from build123d import *

# Parameters (mm, degrees)
BOSS_EXTRUDE1_DEPTH = 4.7625
SKETCH2_R           = 1.25
SKETCH2_W           = 10
SKETCH2_H           = 5
SKETCH2_W_2         = 8
SKETCH2_H_2         = 6
CUT_EXTRUDE1_DEPTH  = 5.7625


with BuildPart() as part:
    # Sketch1 → Boss-Extrude1 (new body)
    with BuildSketch(Plane.XY):
        Polygon((70.6, 40.2), (57.423529412, 29), (0, 29), (0, 0), (84, 0), (100, 29), (100, 40.2), align=None)
    extrude(amount=BOSS_EXTRUDE1_DEPTH)

    # Sketch2 → Cut-Extrude1 (cut, through all)
    with BuildSketch(Plane.XY.offset(4.7625)):
        with Locations((97.2, 37.4)):
            Circle(SKETCH2_R)
        with Locations((75.2, 37.4)):
            Circle(SKETCH2_R)
        with Locations((67.4, 31.1)):
            Circle(SKETCH2_R)
        with Locations((67.4, 9.1)):
            Circle(SKETCH2_R)
        with Locations((75.2, 2.8)):
            Circle(SKETCH2_R)
        with Locations((11, 26.2)):
            Circle(SKETCH2_R)
        with Locations((27, 26.2)):
            Circle(SKETCH2_R)
        with Locations((27, 2.8)):
            Circle(SKETCH2_R)
        with Locations((11, 2.8)):
            Circle(SKETCH2_R)
        with Locations((77.6, 29.7)):
            Rectangle(SKETCH2_W, SKETCH2_H)
        with Locations((77.6, 10.5)):
            Rectangle(SKETCH2_W, SKETCH2_H)
        with Locations((19, 20.5)):
            Rectangle(SKETCH2_W_2, SKETCH2_H_2)
        with Locations((19, 8.5)):
            Rectangle(SKETCH2_W_2, SKETCH2_H_2)
    extrude(amount=-CUT_EXTRUDE1_DEPTH, mode=Mode.SUBTRACT)


solid = part.part
Here's how the part is built. I have some questions about the finished solid (model axes, mm). A direction names the side the tool comes from. Coordinates: 2 decimals unless noted, no trailing zeros. Write each loop counter-clockwise with the first axis right and the second up, starting at its lowest first coordinate (ties: lowest second). Pieces come first, ordered by that corner, then holes. Notation, with made-up numbers: (-30, 37.5) - (-6, 37.5) arc R25 ccw to (-6, 54.5) - close; hole circle Ø11 at (-21.5, -1). An arc over 180 degrees is marked (long way). Use one line per item in the form item = value.
1) I'm going to push flat-ended pins straight in: P1, Ø1.5, axis at x = 75.2, y = 2.8, coming from the +Z side; P2, Ø2.5, axis at y = 10.5, z = 3.5, coming from the +X side; P3, Ø1.4, axis at x = 18.5, z = 2.5, coming from the +Y side. Where does each tip first touch, or does it pass through?
Solved:
P1 = through
P2 = 90.48
P3 = 29
2) Thinking about a two-plate mould opening in X: for faces 4 (the cylindrical face through (10.079, 3.645, 2.415)), 5 (the flat face through (72.6, 30, 2)), 6 (the flat face through (100, 35, 2)), 7 (the flat face through (0, 15, 2)), which applies, released by +X, released by -X, zero draft, split by the parting line, or undercut?
Solved:
face_4 = undercut
face_5 = undercut
face_6 = released by +X
face_7 = released by -X
3) Suppose I cut it at A-A, the plane x = 67.4. Write out the boundary of the cut face in (y, z), plus the area to 3 significant figures.
Solved:
outline = (0, 0) - (7.85, 0) - (7.85, 4.76) - (0, 4.76) - close; (10.35, 0) - (29.85, 0) - (29.85, 4.76) - (10.35, 4.76) - close; (32.35, 0) - (37.48, 0) - (37.48, 4.76) - (32.35, 4.76) - close
area = 155 mm2
4) Suppose I cut it at B-B, the plane z = 2.85. Give the number of separate pieces and of enclosed holes in the cut face, plus the area to 3 significant figures.
Solved:
separate_pieces = 1
enclosed_holes = 13
area = 2,830 mm2
5) On a 3-axis mill with a long thin cutter (end or side, diameter ignored), from which of +Z, -Z, +X, -X, +Y, -Y can I reach the whole of each face in a straight line? I mean faces 1 (the flat face through (82.6, 10, 2)), 2 (the flat face through (29, 29, 2)), 3 (the flat face through (41, 0, 2)). Say none if no direction works.
Solved:
face_1 = +Z, -Z
face_2 = +Z, -Z, -X, +Y
face_3 = +Z, -Z, +X, -X, -Y
6) Suppose I cut it at C-C, the plane y = 9.1. Write out the boundary of the cut face in (x, z), plus the area to 3 significant figures.
Solved:
outline = (0, 0) - (15, 0) - (15, 4.76) - (0, 4.76) - close; (23, 0) - (66.15, 0) - (66.15, 4.76) - (23, 4.76) - close; (68.65, 0) - (72.6, 0) - (72.6, 4.76) - (68.65, 4.76) - close; (82.6, 0) - (89.02, 0) - (89.02, 4.76) - (82.6, 4.76) - close
area = 326 mm2
7) I need wall thicknesses on line 1 (Y direction, x = 81, z = 0.6); line 2 (Y direction, x = 11, z = 2.7); line 3 (Y direction, x = 75.2, z = 2.1). Which ranges of each line are inside material? Lowest first, please.
Solved:
line_1 = 0 to 8, 13 to 27.2, 32.2 to 40.2
line_2 = 0 to 1.55, 4.05 to 24.95, 27.45 to 29
line_3 = 0 to 1.55, 4.05 to 8, 13 to 27.2, 32.2 to 36.15, 38.65 to 40.2
8) Suppose I cut it at D-D, the plane y = 37.4. Write out the boundary of the cut face in (x, z), plus the area to 3 significant figures.
Solved:
outline = (67.31, 0) - (73.95, 0) - (73.95, 4.76) - (67.31, 4.76) - close; (76.45, 0) - (95.95, 0) - (95.95, 4.76) - (76.45, 4.76) - close; (98.45, 0) - (100, 0) - (100, 4.76) - (98.45, 4.76) - close
area = 132 mm2
